The listing builds one solid part. Answer for the finished solid, in the listing's coordinates (mm). Coordinates: 2 decimals unless noted, no trailing zeros. Loops run counter-clockwise (first coordinate to the right, second up) from the corner with the lowest first, then second, coordinate; pieces in that order, holes last. Notation, with made-up numbers: (-37, -21) - (21, -21) arc R24 cw to (21, 7) - close; hole circle Ø8 at (-33.5, 30.25). An arc over 180 degrees is marked (long way). Write each question's results on one line, items separated by ' | '. Start each with the question number.
(1) Consider line 1 (Y direction, x = 73.5, z = 0.8); line 2 (X direction, y = -13, z = 1.75); line 3 (Y direction, x = 4, z = 2.15). Determine where each line is inside the solid, lowest interval first. Write a range as from..to.
(2) Find section C-C on z = 1.95. State how many separate pieces and enclosed holes the cut face has, then the cut area to 3 significant figures.
(3) Find section B-B on x = -26.5. Determine the outline of the cut face in (y, z), then the cut area to 3 significant figures.
(4) Given pin 1 Ø2 at (y, z) = (-62, 2.5) entering from -X; pin 2 Ø2 at (x, z) = (29.5, 2.5) entering from -Y, each flat-ended and moving along its own axis, determine where each tip first touches the part or whether it passes through.
(5) Find section A-A on x = -48. Determine the outline of the cut face in (y, z).
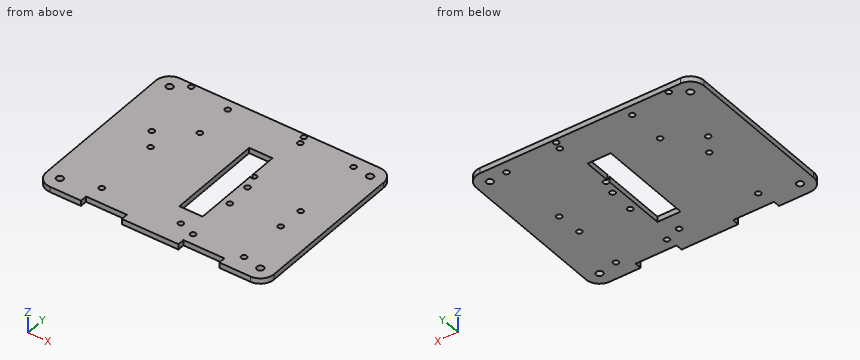
from build123d import *

# Parameters (mm, degrees)
SKETCH1_W           = 167
SKETCH1_H           = 130
BOSS_EXTRUDE1_DEPTH = 4
FILLET1_R           = 10
FILLET2_R           = 10
SKETCH5_R           = 2.5
CUT_EXTRUDE4_DEPTH  = 70
SKETCH6_W           = 30
SKETCH6_H           = 5
CUT_EXTRUDE5_DEPTH  = 10
SKETCH7_R           = 2
CUT_EXTRUDE6_DEPTH  = 106.892634305
SKETCH8_R           = 2
CUT_EXTRUDE7_DEPTH  = 106.892634305
SKETCH9_W           = 17
SKETCH9_H           = 70
CUT_EXTRUDE8_DEPTH  = 106.892634305
SKETCH10_R          = 2
CUT_EXTRUDE9_DEPTH  = 106.892634305
SKETCH11_R          = 2
CUT_EXTRUDE10_DEPTH = 106.892634305


with BuildPart() as part:
    # Sketch1 → Boss-Extrude1 (new body)
    with BuildSketch(Plane.XY):
        Rectangle(SKETCH1_W, SKETCH1_H)
    extrude(amount=BOSS_EXTRUDE1_DEPTH)

    # Fillet1
    fillet1_edges = [part.edges().sort_by_distance(p)[0] for p in [
        (-83.5, -65, 2),
        (-83.5, 65, 2),
    ]]
    fillet(fillet1_edges, radius=FILLET1_R)

    # Fillet2
    fillet2_edges = [part.edges().sort_by_distance(p)[0] for p in [
        (83.5, -65, 2),
        (83.5, 65, 2),
    ]]
    fillet(fillet2_edges, radius=FILLET2_R)

    # Sketch5 → Cut-Extrude4 (cut)
    with BuildSketch(Plane.XY.offset(4)):
        with Locations((-73.5, 55)):
            Circle(SKETCH5_R)
        with Locations((73.5, 55)):
            Circle(SKETCH5_R)
        with Locations((-73.5, -55)):
            Circle(SKETCH5_R)
        with Locations((73.5, -55)):
            Circle(SKETCH5_R)
    extrude(amount=-CUT_EXTRUDE4_DEPTH, mode=Mode.SUBTRACT)

    # Sketch6 → Cut-Extrude5 (cut)
    with BuildSketch(Plane.XY.offset(4)):
        with Locations((-35.714992286, -62.5)):
            Rectangle(SKETCH6_W, SKETCH6_H)
        with Locations((35.714992286, -62.5)):
            Rectangle(SKETCH6_W, SKETCH6_H)
    extrude(amount=-CUT_EXTRUDE5_DEPTH, mode=Mode.SUBTRACT)

    # Sketch7 → Cut-Extrude6 (cut, through all)
    with BuildSketch(Plane.XY.offset(4)):
        with Locations((22.006812394, -15.314288265)):
            Circle(SKETCH7_R)
        with Locations((59.386313266, -15.314288265)):
            Circle(SKETCH7_R)
        with Locations((59.386313266, -52.056088589)):
            Circle(SKETCH7_R)
        with Locations((22.006812394, -52.056088589)):
            Circle(SKETCH7_R)
    extrude(amount=-CUT_EXTRUDE6_DEPTH, mode=Mode.SUBTRACT)

    # Sketch8 → Cut-Extrude7 (cut, through all)
    with BuildSketch(Plane.XY.offset(4)):
        with Locations((21.25, 56.5)):
            Circle(SKETCH8_R)
        with Locations((60.25, 56.5)):
            Circle(SKETCH8_R)
        with Locations((60.25, 3.5)):
            Circle(SKETCH8_R)
        with Locations((21.25, 3.5)):
            Circle(SKETCH8_R)
    extrude(amount=-CUT_EXTRUDE7_DEPTH, mode=Mode.SUBTRACT)

    # Sketch9 → Cut-Extrude8 (cut, through all)
    with BuildSketch(Plane.XY.offset(4)):
        with Locations((8, 0)):
            Rectangle(SKETCH9_W, SKETCH9_H)
    extrude(amount=-CUT_EXTRUDE8_DEPTH, mode=Mode.SUBTRACT)

    # Sketch10 → Cut-Extrude9 (cut, through all)
    with BuildSketch(Plane.XY.offset(4)):
        with Locations((-48, 1.082115111)):
            Circle(SKETCH10_R)
        with Locations((10, -47.917884889)):
            Circle(SKETCH10_R)
        with Locations((-48, -47.917884889)):
            Circle(SKETCH10_R)
        with Locations((10, 1.082115111)):
            Circle(SKETCH10_R)
    extrude(amount=-CUT_EXTRUDE9_DEPTH, mode=Mode.SUBTRACT)

    # Sketch11 → Cut-Extrude10 (cut, through all)
    with BuildSketch(Plane.XY.offset(4)):
        with Locations((-63.02, 62.378539804)):
            Circle(SKETCH11_R)
        with Locations((-32.54, 57.298539804)):
            Circle(SKETCH11_R)
        with Locations((-32.54, 29.358539804)):
            Circle(SKETCH11_R)
        with Locations((19.53, 62.378539804)):
            Circle(SKETCH11_R)
        with Locations((18.26, 14.118539804)):
            Circle(SKETCH11_R)
        with Locations((-56.67, 14.118539804)):
            Circle(SKETCH11_R)
    extrude(amount=-CUT_EXTRUDE10_DEPTH, mode=Mode.SUBTRACT)


solid = part.part
Values:
1) line 1: y = -65..-57.5, -52.5..52.5, 57.5..65 | line 2: x = -83.5..-0.5, 16.5..83.5 | line 3: y = -65..-35, 35..65
2) separate pieces: 1 | enclosed holes: 21 | area: 19,800 mm²
3) outline: (-60, 0) - (65, 0) - (65, 4) - (-60, 4) - close | area: 500 mm²
4) pin 1: stops at x = -81.5 | pin 2: stops at y = -60
5) outline: (-60, 0) - (-49.92, 0) - (-49.92, 4) - (-60, 4) - close; (-45.92, 0) - (-0.92, 0) - (-0.92, 4) - (-45.92, 4) - close; (3.08, 0) - (65, 0) - (65, 4) - (3.08, 4) - close
